from build123d import *

# Parameters (mm, degrees)
CROQUIS1_W              = 3.5
CROQUIS1_H              = 3.5
SALIENTE_EXTRUIR1_DEPTH = 15
CROQUIS4_W              = 4.7
CROQUIS4_H              = 10
SALIENTE_EXTRUIR2_DEPTH = 0.5
CROQUIS5_W              = 2.5
CROQUIS5_H              = 2.5
CORTAR_EXTRUIR1_DEPTH   = 14


with BuildPart() as part:
    # Croquis1 → Saliente-Extruir1 (new body)
    with BuildSketch(Plane(origin=(0, 0, 0), x_dir=(0, 0, -1), z_dir=(1, 0, 0))):
        with Locations((0, 1.75)):
            Rectangle(CROQUIS1_W, CROQUIS1_H)
    extrude(amount=SALIENTE_EXTRUIR1_DEPTH)

    # Croquis4 → Saliente-Extruir2 (add)
    with BuildSketch(Plane.ZY.offset(-5.15)):
        with Locations((0, 1.75)):
            Rectangle(CROQUIS4_W, CROQUIS4_H)
    extrude(amount=-SALIENTE_EXTRUIR2_DEPTH)

    # Croquis5 → Cortar-Extruir1 (cut)
    with BuildSketch(Plane(origin=(15, 0, 0), x_dir=(0, 0, -1), z_dir=(1, 0, 0))):
        with Locations((0, 1.75)):
            Rectangle(CROQUIS5_W, CROQUIS5_H)
    extrude(amount=-CORTAR_EXTRUIR1_DEPTH, mode=Mode.SUBTRACT)


solid = part.part
Verification items for the finished model (mm, model axes). A direction names the side the tool comes from. Coordinates: 2 decimals unless noted, no trailing zeros. Write each loop counter-clockwise with the first axis right and the second up, starting at its lowest first coordinate (ties: lowest second). Pieces come first, ordered by that corner, then holes. Notation, with made-up numbers: (81, 60.5) - (103, 60.5) arc R11 ccw to (103, 75.5) - close; hole circle Ø7 at (-21.75, 50). An arc over 180 degrees is marked (long way). Answer as a JSON object with one key per item and string values.
(1) Cross-section at C-C on y = -1.75. Record the cut outline in (x, z).
Report:
{"outline": "(5.15, -2.35) - (5.65, -2.35) - (5.65, 2.35) - (5.15, 2.35) - close"}
(2) Mould release check, pull along Y, two halves, no side actions. Record for faces 5 (the flat face through (10, 0, 0)), 6 (the flat face through (8, 2, 1.25)), 7 (the flat face through (1, 2, 0)), 8 (the flat face through (5.15, 2, -2)): pulls with the +Y half, pulls with the -Y half, needs draft (parallel to the pull), parting line crosses it, or undercut.
Report:
{"face 5": "pulls with the -Y half", "face 6": "undercut", "face 7": "undercut", "face 8": "needs draft"}
(3) Cross-section at A-A on x = 9. Record the cut outline in (y, z), plus the area to 3 significant figures.
Report:
{"outline": "(0, -1.75) - (3.5, -1.75) - (3.5, 1.75) - (0, 1.75) - close; hole (0.5, -1.25) - (3, -1.25) - (3, 1.25) - (0.5, 1.25) - close", "area": "6.00 mm^2"}
(4) Gauge pin test, flat ends, axial feed: pin 1 Ø6 at (x, y) = (5, 1) entering from -Z; pin 2 Ø1.8 at (x, y) = (10.5, 1.5) entering from +Z; pin 3 Ø1.2 at (x, z) = (9, 0) entering from +Y; pin 4 Ø3 at (x, y) = (2, 2) entering from -Z. Record the tip position at first contact, or that the pin passes through.
Report:
{"pin 1": "z = -2.35", "pin 2": "z = 1.75", "pin 3": "y = 3.5", "pin 4": "z = -1.75"}
(5) Thickness scan on line 1 along Y through (x, z) = (5.5, -0.5); line 2 along Y through (x, z) = (10, 0.55); line 3 along X through (y, z) = (3.75, -0.7). Record the ranges inside material, lowest first.
Report:
{"line 1": "-3.25 to 0.5, 3 to 6.75", "line 2": "0 to 0.5, 3 to 3.5", "line 3": "5.15 to 5.65"}
(6) Cross-section at D-D on z = 1.55. Record the cut outline in (x, y), plus the area to 4 significant figures.
Report:
{"outline": "(0, 0) - (5.15, 0) - (5.15, -3.25) - (5.65, -3.25) - (5.65, 0) - (15, 0) - (15, 3.5) - (5.65, 3.5) - (5.65, 6.75) - (5.15, 6.75) - (5.15, 3.5) - (0, 3.5) - close", "area": "55.75 mm^2"}
(7) Tool access check on faces 1 (the flat face through (10, 2, -1.75)), 2 (the flat face through (3, 2, -1.75)), 3 (the flat face through (8, 3, 0)), 4 (the flat face through (10, 3.5, 0)). Record the directions out of +Z, -Z, +X, -X, +Y, -Y that give a thin tool (end or side, any length) a straight path to the whole face; none if there is none.
Report:
{"face 1": "-Z, +X, +Y, -Y", "face 2": "-Z, -X, +Y, -Y", "face 3": "+X", "face 4": "+Z, -Z, +X, +Y"}
(8) Cross-section at B-B on z = 0.4. Record the cut outline in (x, y).
Report:
{"outline": "(0, 0) - (5.15, 0) - (5.15, -3.25) - (5.65, -3.25) - (5.65, 0) - (15, 0) - (15, 0.5) - (1, 0.5) - (1, 3) - (15, 3) - (15, 3.5) - (5.65, 3.5) - (5.65, 6.75) - (5.15, 6.75) - (5.15, 3.5) - (0, 3.5) - close"}
